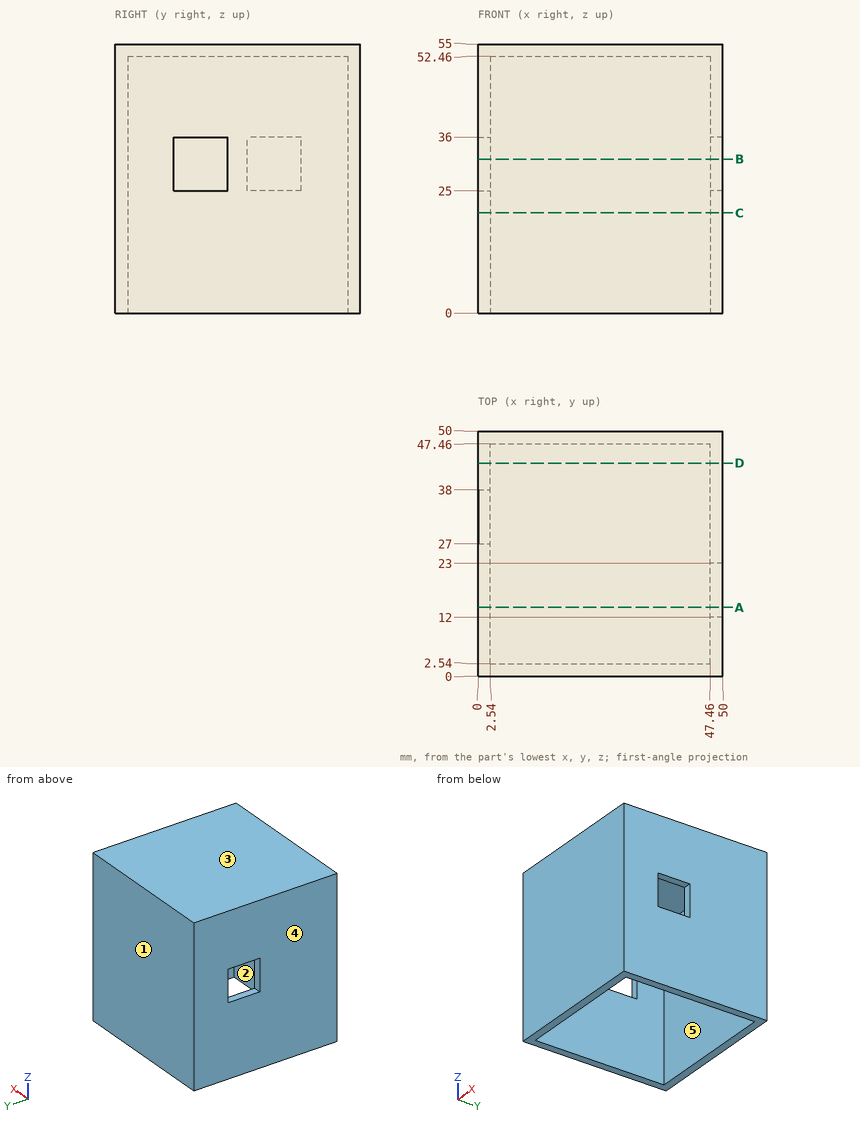
Geometry: see drawing. Coordinates: mm, zero at the bounding-box minimum. A direction names the side the tool comes from. Coordinates: 2 decimals unless noted, no trailing zeros. Loops run counter-clockwise (first coordinate to the right, second up) from the corner with the lowest first, then second, coordinate; pieces in that order, holes last. Notation, with made-up numbers: (60, -11.75) - (70, -11.75) arc R32 ccw to (70, 20.25) - close; hole circle Ø1 at (-13.5, -12.75). An arc over 180 degrees is marked (long way). Answer in a Markdown table with one row per item.
(1) Material intervals for L1, parallel to X at y = 11.5, z = 26; L2, parallel to Z at x = 28, y = 16.5, sorted ascending. Write a range as from..to.
Model answer:
| item | result |
|---|---|
| L1 | x = 0..2.54, 47.46..50 |
| L2 | z = 52.46..55 |
(2) Cut plane B-B on z = 31.5. Output: boundary loops of the cut face in (x, y), plus the area to 3 significant figures.
Model answer:
| item | result |
|---|---|
| outline | (0, 0) - (50, 0) - (50, 12) - (47.46, 12) - (47.46, 2.54) - (2.54, 2.54) - (2.54, 27) - (0, 27) - close; (0, 38) - (2.54, 38) - (2.54, 47.46) - (47.46, 47.46) - (47.46, 23) - (50, 23) - (50, 50) - (0, 50) - close |
| area | 426 mm² |
(3) Cut plane D-D on y = 43.5. Output: boundary loops of the cut face in (x, z), plus the area to 3 significant figures.
Model answer:
| item | result |
|---|---|
| outline | (0, 0) - (2.54, 0) - (2.54, 52.46) - (47.46, 52.46) - (47.46, 0) - (50, 0) - (50, 55) - (0, 55) - close |
| area | 393 mm² |
(4) Cut plane A-A on y = 14. Output: boundary loops of the cut face in (x, z).
Model answer:
| item | result |
|---|---|
| outline | (0, 0) - (2.54, 0) - (2.54, 52.46) - (47.46, 52.46) - (47.46, 36) - (50, 36) - (50, 55) - (0, 55) - close; (47.46, 0) - (50, 0) - (50, 25) - (47.46, 25) - close |
(5) Mould query, pull axis Y, two halves, no side actions, for the marked faces 1, 2 and 3. Classes: pulls with the +Y half, pulls with the -Y half, needs draft (parallel to the pull), parting line crosses it, or undercut.
Model answer:
| item | result |
|---|---|
| face 1 | pulls with the +Y half |
| face 2 | undercut |
| face 3 | needs draft |
(6) Set-up query: the marked faces 4 and 5. Return all of +Z, -Z, +X, -X, +Y, -Y with unobstructed straight access to the full face (end or side cutting, diameter ignored); none if empty.
Model answer:
| item | result |
|---|---|
| face 4 | +Z, -Z, -X, +Y, -Y |
| face 5 | -Z |
(7) Pin query (flat end, axial travel): P1, Ø2, axis at y = 25.5, z = 17, coming from the -X side; P2, Ø13.5, axis at x = 24, y = 27, coming from the -Z side. Return the tip coordinate at first contact, or that it passes through.
Model answer:
| item | result |
|---|---|
| P1 | stops at x = 0 |
| P2 | stops at z = 52.46 |
(8) Cut plane C-C on z = 20.5. Output: boundary loops of the cut face in (x, y).
Model answer:
| item | result |
|---|---|
| outline | (0, 0) - (50, 0) - (50, 50) - (0, 50) - close; hole (2.54, 2.54) - (47.46, 2.54) - (47.46, 47.46) - (2.54, 47.46) - close |
